Could you check a few things on this drawing? It's one solid part, dimensions in mm from its lowest x, y, z. A direction names the side the tool comes from. Give positions to 0.01 mm unless a question says otherwise; leave off trailing zeros. Order: outer loops, then holes, each group sorted by start corner. A loop starts at its lowest first (then second) coordinate and runs counter-clockwise, first axis right, second up. Notation, with made-up numbers: (-28, -16) - (-17, -16) arc R20 ccw to (-17, 11) - close; hole circle Ø9 at (-20.75, -24.75). An arc over 180 degrees is marked (long way). Return JSON: item names as keys, results as strings.
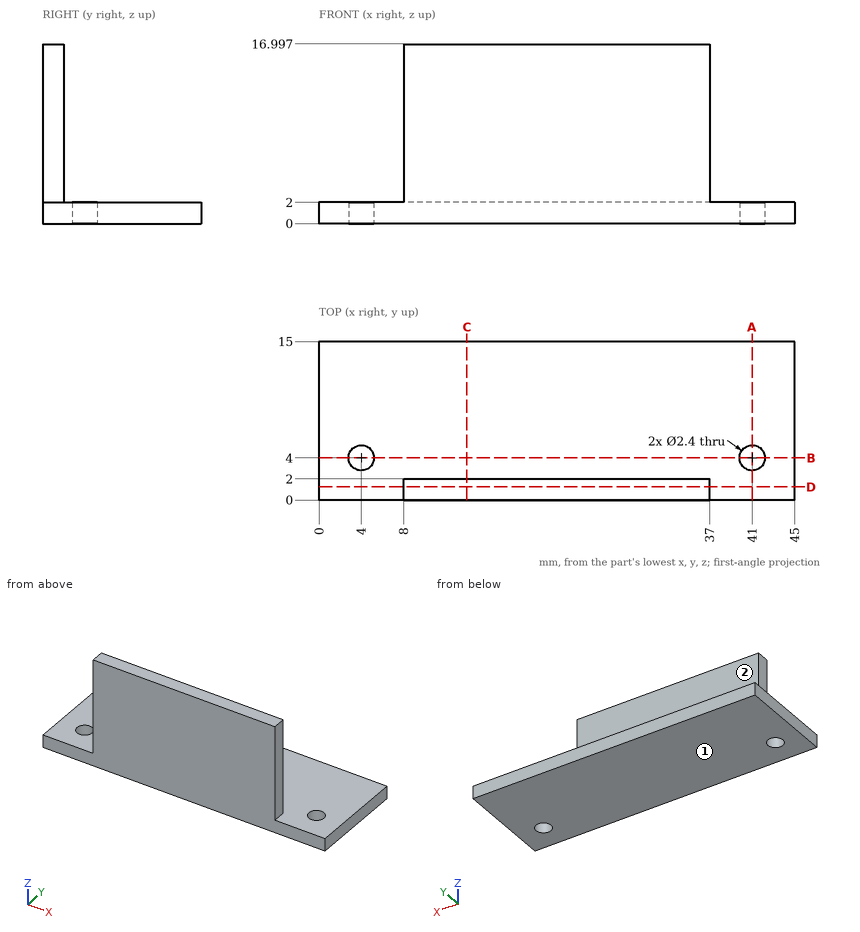
1. Suppose I cut it at B-B (y = 4). List the corners of the cut face in (x, z) for me.
Checks:
{"outline": "(0, 0) - (2.8, 0) - (2.8, 2) - (0, 2) - close; (5.2, 0) - (39.8, 0) - (39.8, 2) - (5.2, 2) - close; (42.2, 0) - (45, 0) - (45, 2) - (42.2, 2) - close"}
2. On a 3-axis mill with a long thin cutter (end or side, diameter ignored), from which of +Z, -Z, +X, -X, +Y, -Y can I reach the whole of each face in a straight line? I mean the marked faces 1 and 2. Say none if no direction works.
Checks:
{"face 1": "-Z, +X, -X, +Y, -Y", "face 2": "+Z, +X, -X, +Y"}
3. Suppose I cut it at C-C (x = 14). List the corners of the cut face in (y, z) for me.
Checks:
{"outline": "(0, 0) - (15, 0) - (15, 2) - (2, 2) - (2, 17) - (0, 17) - close"}
4. For pin 1 Ø2 at (y, z) = (1.5, 12) entering from +X; pin 2 Ø4 at (x, y) = (23, 8.5) entering from +Z; pin 3 Ø4 at (x, z) = (25.5, 13.5) entering from +Y, each with a flat end and sliding along its axis, tell me the tip position at first contact or that it passes through.
Checks:
{"pin 1": "x = 37", "pin 2": "z = 2", "pin 3": "y = 2"}
5. If I drill on L1, parallel to Y at x = 41, z = 1.45; L2, parallel to Z at x = 10.5, y = 11.25, over which ranges is the centre line in solid material (lowest first)? Write a range as [from, to].
Checks:
{"L1": "[0, 2.8], [5.2, 15]", "L2": "[0, 2]"}
6. Suppose I cut it at D-D (y = 1.25). List the corners of the cut face in (x, z) for me.
Checks:
{"outline": "(0, 0) - (45, 0) - (45, 2) - (37, 2) - (37, 17) - (8, 17) - (8, 2) - (0, 2) - close"}
7. Suppose I cut it at A-A (x = 41). List the corners of the cut face in (y, z) for me, plus the area to 3 significant figures.
Checks:
{"outline": "(0, 0) - (2.8, 0) - (2.8, 2) - (0, 2) - close; (5.2, 0) - (15, 0) - (15, 2) - (5.2, 2) - close", "area": "25.2 mm^2"}
